Autodesk Inventor part; units mm, degrees
ref_plane "YZ Plane" through (0, 0, 0) normal (1, 0, 0) x (0, 1, 0)
ref_plane "XZ Plane" through (0, 0, 0) normal (0, 1, 0) x (-1, 0, 0)
ref_plane "XY Plane" through (0, 0, 0) normal (0, 0, 1) x (1, 0, 0)
sketch "草圖1" plane through (0, 0, 0) normal (0, 1, 0) x (-1, 0, 0)
  line L0 (12.5, 7.5) -> (-12.5, 7.5)
  line L1 (-12.5, 7.5) -> (-12.5, -7.5)
  line L2 (-12.5, -7.5) -> (12.5, -7.5)
  line L3 (12.5, -7.5) -> (12.5, 7.5)
  line L4 (12.5, 7.5) -> (-12.5, -7.5) construction
  line L5 (-12.5, 7.5) -> (12.5, -7.5) construction
  point P0 (0, 0)
  dimension "d0" = 25
  dimension "d1" = 15
extrude "擠出1" add sketch "草圖1" along normal blind 75 draft -2
sketch "草圖2" plane through (0, 75, 0) normal (0, 1, 0) x (1, 0, 0)
  line L0 (9.8809, -4.8809) -> (-9.8809, -4.8809)
  line L1 (9.8809, 4.8809) -> (9.8809, -4.8809)
  line L2 (-9.8809, 4.8809) -> (9.8809, 4.8809)
  line L3 (-9.8809, -4.8809) -> (-9.8809, 4.8809)
  point P0 (0, 0)
extrude "擠出2" add sketch "草圖2" along normal blind 15
sketch "草圖3" plane through (9.8809, 75, -4.8809) normal (0, 0, -1) x (-1, 0, 0)
  line L0 (19.7619, 0) -> (0, 0)
  line L1 (19.7619, 0) -> (19.7619, 15)
  line L2 (0, 15) -> (19.7619, 15)
  line L3 (0, 0) -> (0, 15)
  line L4 (0, 15) -> (19.7619, 15)
  line L5 (5.1309, 15) -> (14.6309, 15)
  line L6 (14.6309, 15) -> (14.6309, 8)
  line L7 (14.6309, 8) -> (5.1309, 8)
  line L8 (5.1309, 8) -> (5.1309, 15)
  point P0 (9.8809, -75)
  point P1 (9.8809, 8)
  point P2 (9.8809, 15)
  dimension "d6" = 9.5
  dimension "d7" = 7
hole "孔1" at (4.75, 83, -4.8809) at (-4.75, 83, -4.8809) direction (0, 0, 1) diameter 2 end through all counterbore diameter 3.25 counterbore depth 5.8
sketch "草圖4" plane through (0, 0, 0) normal (0, -1, 0) x (1, 0, 0)
  point P0 (0, 0)
  point P1 (5, 0)
  point P2 (-5, 0)
  dimension "d15" = 10
  dimension "d16" = 5
hole "孔2" at (5, 0, 0) at (-5, 0, 0) direction (0, 1, 0) diameter 2.7 depth 20 counterbore diameter 4.1 counterbore depth 6
properties part number "限位開關架"
Input: part model. Units: mm. Frame: model coordinates. A direction names the side the tool comes from. Coordinates: 2 decimals unless noted, no trailing zeros. Order: outer loops, then holes, each group sorted by start corner. A loop starts at its lowest first (then second) coordinate and runs counter-clockwise, first axis right, second up. Notation, with made-up numbers: (-17.75, -3.75) - (-7.75, -3.75) arc R14 ccw to (-7.75, 2.25) - close; hole circle Ø11 at (-9, 28). An arc over 180 degrees is marked (long way). Return JSON: item names as keys, results as strings.
Q1. Ray query, probe 1 along X at (y, z) = (83, -3.3) (3 decimals); probe 2 along Y at (x, z) = (4.75, -3.2) (3 decimals); probe 3 along Y at (x, z) = (-4.75, 2.6). Return the intervals inside material, ascending.
The answers:
{"probe 1": "x = -9.881 to -6.375, -3.125 to 3.125, 6.375 to 9.881", "probe 2": "y = 0 to 81.375, 84.625 to 90", "probe 3": "y = 0 to 82, 84 to 90"}
Q2. Cut plane C-C (y = 10). Return loops of the section in (x, z).
The answers:
{"outline": "(-12.15, -7.15) - (12.15, -7.15) - (12.15, 7.15) - (-12.15, 7.15) - close; hole circle Ø2.7 at (-5, 0); hole circle Ø2.7 at (5, 0)"}
Q3. Access query for faces 1 (the cylindrical face through (-2.999, 3.042, 0.444)), 2 (the flat face through (0, 82, 4.881)), 3 (the flat face through (0, 82, -4.881)), 4 (the cylindrical face through (-5.24, 84.55, -1.94)). Directions: +Z, -Z, +X, -X, +Y, -Y. A direction counts if a zero-diameter tool reaches every point of the face in a straight line with its end or side. Return the directions, or none.
The answers:
{"face 1": "-Y", "face 2": "+Z, +X, -X, +Y", "face 3": "-Z, +X, -X, +Y", "face 4": "-Z"}
Q4. Cut plane A-A (y = 83). Return loops of the section in (x, z) (3 decimals).
The answers:
{"outline": "(-9.881, -4.881) - (-6.375, -4.881) - (-6.375, 0.919) - (-5.75, 0.919) - (-5.75, 4.881) - (-9.881, 4.881) - close; (-3.75, 0.919) - (-3.125, 0.919) - (-3.125, -4.881) - (3.125, -4.881) - (3.125, 0.919) - (3.75, 0.919) - (3.75, 4.881) - (-3.75, 4.881) - close; (5.75, 0.919) - (6.375, 0.919) - (6.375, -4.881) - (9.881, -4.881) - (9.881, 4.881) - (5.75, 4.881) - close"}
Q5. Cut plane B-B (z = 0). State how many separate pieces and enclosed holes the cut face has, then the cut area to 3 significant figures.
The answers:
{"separate pieces": "1", "enclosed holes": "2", "area": "1,830 mm2"}
Q6. Draft query along Y for faces 5 (the flat face through (0, 0, 0)), 6 (the cylindrical face through (4.7, 82, 2.9)), 7 (the cylindrical face through (7.001, 3.042, 0.444)). Return one class per face: +Y half, -Y half, draft (parallel to the pull), parting line (faces both ways), or undercut.
The answers:
{"face 5": "-Y half", "face 6": "undercut", "face 7": "draft"}
Q7. First-contact query: pin 1 (0.8 mm diameter, centred on x = -4.5, z = -0.5, fed in from -Y); pin 2 (4 mm diameter, centred on y = 50.5, z = -3, fed in from +X); pin 3 (4.5 mm diameter, centred on x = -5, y = 84, fed in from -Z). Flat tips, straight axial feed; report the tip coordinate or a pass-through.
The answers:
{"pin 1": "stops at y = 20", "pin 2": "stops at x = 10.81", "pin 3": "stops at z = -4.88"}
Q8. Cut plane D-D (z = -6.5). Return loops of the section in (x, y).
The answers:
{"outline": "(-12.5, 0) - (12.5, 0) - (11.5, 28.64) - (-11.5, 28.64) - close"}
